Can you work these out from the drawing? Everything is in mm from the part's minimum corner. Round coordinates to 2 decimals unless told otherwise and drop trailing zeros. Write each loop counter-clockwise with the first axis right and the second up, starting at its lowest first coordinate (ties: lowest second). Pieces come first, ordered by that corner, then holes. Notation, with made-up numbers: (10, 2) -> (49, 2) arc R14 ccw to (49, 26) -> close; hole circle Ø2 at (75.25, 62.5). An arc over 180 degrees is marked (long way). One line per question, with ' | ' between items. Start each with the question number.
1. Imagine slicing it at A-A, the plane x = 4. List the corners of the cut face in (y, z) for me.
2. Imagine slicing it at B-B, the plane z = 4. List the corners of the cut face in (x, y) for me, and give its area (3 significant figures).
3. Thinking about a two-plate mould opening in Z: for the marked faces 1, 2 and 3, which applies, released by +Z, released by -Z, zero draft, split by the parting line, or undercut?
4. Imagine slicing it at D-D, the plane x = 6.5. List the corners of the cut face in (y, z) for me.
5. If I drill on line 1 along Z through (x, y) = (4, 5.5); line 2 along X through (y, z) = (1, 3.5), over which ranges is the centre line in solid material (lowest first)? Write a range as [from, to].
6. Imagine slicing it at C-C, the plane y = 3. List the corners of the cut face in (x, z) for me.
7. For pin 1 Ø1.9 at (x, z) = (4, 4) entering from +Y; pin 2 Ø1.5 at (y, z) = (5, 1) entering from +X, each with a flat end and sliding along its axis, tell me the tip position at first contact or that it passes through.
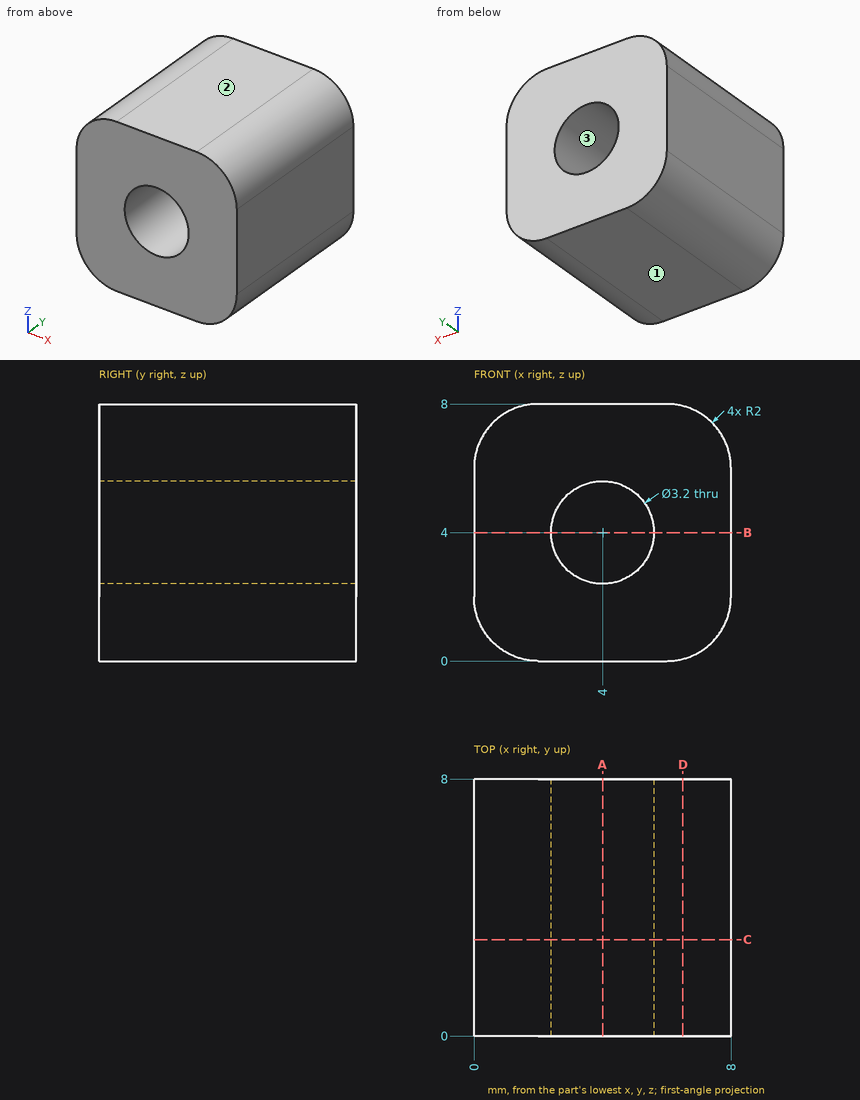
Geometry results:
1) outline: (0, 0) -> (8, 0) -> (8, 2.4) -> (0, 2.4) -> close; (0, 5.6) -> (8, 5.6) -> (8, 8) -> (0, 8) -> close
2) outline: (0, 0) -> (2.4, 0) -> (2.4, 8) -> (0, 8) -> close; (5.6, 0) -> (8, 0) -> (8, 8) -> (5.6, 8) -> close | area: 38.4 mm2
3) face 1: released by -Z | face 2: released by +Z | face 3: undercut
4) outline: (0, 0.06) -> (8, 0.06) -> (8, 7.94) -> (0, 7.94) -> close
5) line 1: z = [0, 2.4], [5.6, 8] | line 2: x = [0, 2.48], [5.52, 8]
6) outline: (0, 2) arc R2 ccw to (2, 0) -> (6, 0) arc R2 ccw to (8, 2) -> (8, 6) arc R2 ccw to (6, 8) -> (2, 8) arc R2 ccw to (0, 6) -> close; hole circle Ø3.2 at (4, 4)
7) pin 1: passes through | pin 2: stops at x = 7.98
